Input: part model. Units: mm. Frame: model coordinates. A direction names the side the tool comes from. Coordinates: 2 decimals unless noted, no trailing zeros. Loops run counter-clockwise (first coordinate to the right, second up) from the corner with the lowest first, then second, coordinate; pieces in that order, holes last. Notation, with made-up numbers: M 15,82.25 L 31,82.25 A24 ccw 31,93.25 Z; hole C -4,19 d4. An arc over 180 degrees is marked long. Use a Markdown table: item, result. Add a question column.
1. Pin query (flat end, axial travel): pin 1 (3 mm diameter, centred on y = 5, z = 2, fed in from +X); pin 2 (5 mm diameter, centred on x = -1.5, z = 7, fed in from -Y); pin 3 (1 mm diameter, centred on y = -3, z = 4, fed in from +X); pin 4 (1.5 mm diameter, centred on x = -0.5, y = 0, fed in from +Z). Return the tip coordinate at first contact, or that it passes through.
2. Set-up query: faces 1 (the flat face through (2, -2, 11.2)), 2 (the cylindrical face through (-6, 0, 5)). Return all of +Z, -Z, +X, -X, +Y, -Y with unobstructed straight access to the full face (end or side cutting, diameter ignored); none if empty.
3. Section D-D on y = 5.75. Output: boundary loops of the cut face in (x, z).
4. Section A-A on y = 0. Output: boundary loops of the cut face in (x, z), then the cut area to 3 significant figures.
5. Line query: L1, parallel to Z at x = -6.25, y = 3.5; L2, parallel to Y at x = 0, z = 7.75; L3, parallel to Y at x = -0.75, z = 6. Output: solid intervals per line, ascending. Write a range as [from, to].
6. Section C-C on z = 4.5. Output: boundary loops of the cut face in (x, y), then the cut area to 3 significant figures.
```python
from build123d import *

# Parameters (mm, degrees)
F0_R     = 6
F1_DEPTH = 10
F2_R     = 7.25
F2_R_2   = 6
F3_DEPTH = 1.2
F4_R     = 2
F5_DEPTH = 25


with BuildPart() as f1:
    # F0 (on Top) → F1 (new body)
    with BuildSketch(Plane.XY):
        Circle(F0_R)
    extrude(amount=F1_DEPTH)

    # F2 (on face) → F3 (join)
    with BuildSketch(Plane.XY.offset(10)):
        Circle(F2_R)
        Circle(F2_R_2, mode=Mode.SUBTRACT)
        Circle(F2_R_2)
    extrude(amount=F3_DEPTH)

    # F4 (on face) → F5 (cut)
    with BuildSketch(Plane.XY.offset(11.2)):
        Circle(F4_R)
    extrude(amount=-F5_DEPTH, mode=Mode.SUBTRACT)


solid = f1.part
```
Answers below:
| question | item | result |
|---|---|---|
| 1 | pin 1 | stops at x = 4.87 |
| 1 | pin 2 | stops at y = -6 |
| 1 | pin 3 | stops at x = 5.45 |
| 1 | pin 4 | passes through |
| 2 | face 1 | +Z, +X, -X, +Y, -Y |
| 2 | face 2 | -Z |
| 3 | outline | M -4.42,10 L -1.71,10 L -1.71,0 L 1.71,0 L 1.71,10 L 4.42,10 L 4.42,11.2 L -4.42,11.2 Z |
| 4 | outline | M -7.25,10 L -6,10 L -6,0 L -2,0 L -2,11.2 L -7.25,11.2 Z; M 2,0 L 6,0 L 6,10 L 7.25,10 L 7.25,11.2 L 2,11.2 Z |
| 4 | area | 92.6 mm² |
| 5 | L1 | z = [10, 11.2] |
| 5 | L2 | y = [-6, -2], [2, 6] |
| 5 | L3 | y = [-5.95, -1.85], [1.85, 5.95] |
| 6 | outline | C 0,0 d12; hole C 0,0 d4 |
| 6 | area | 101 mm² |
